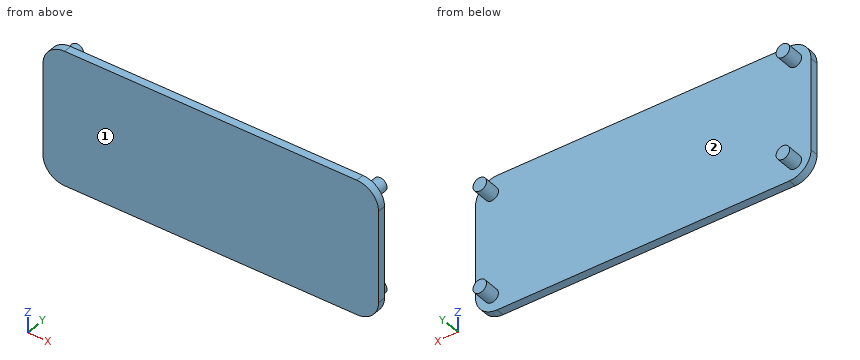
from build123d import *

# Parameters (mm, degrees)
CROQUIS1_W              = 62
CROQUIS1_H              = 25
SALIENTE_EXTRUIR1_DEPTH = 1.5
REDONDEO1_R             = 4
CROQUIS2_R              = 1.25
SALIENTE_EXTRUIR2_DEPTH = 3


with BuildPart() as part:
    # Croquis1 → Saliente-Extruir1 (new body)
    with BuildSketch(Plane(origin=(0, 0, 0), x_dir=(1, 0, 0), z_dir=(0, 1, 0))):
        Rectangle(CROQUIS1_W, CROQUIS1_H)
    extrude(amount=SALIENTE_EXTRUIR1_DEPTH)

    # Redondeo1
    redondeo1_edges = [part.edges().sort_by_distance(p)[0] for p in [
        (31, 0.75, 12.5),
        (-31, 0.75, 12.5),
        (-31, 0.75, -12.5),
        (31, 0.75, -12.5),
    ]]
    fillet(redondeo1_edges, radius=REDONDEO1_R)

    # Croquis2 → Saliente-Extruir2 (add)
    with BuildSketch(Plane(origin=(0, 1.5, 0), x_dir=(1, 0, 0), z_dir=(0, 1, 0))):
        with Locations((-28, 9.47)):
            Circle(CROQUIS2_R)
        with Locations((28, 9.47)):
            Circle(CROQUIS2_R)
        with Locations((28, -9.47)):
            Circle(CROQUIS2_R)
        with Locations((-28, -9.47)):
            Circle(CROQUIS2_R)
    extrude(amount=SALIENTE_EXTRUIR2_DEPTH)


solid = part.part
Model file for the job. Use its own axes, mm. Face numbers are marked on the shaded views. Coordinates: 2 decimals unless noted, no trailing zeros. Order: outer loops, then holes, each group sorted by start corner. A loop starts at its lowest first (then second) coordinate and runs counter-clockwise, first axis right, second up. Notation, with made-up numbers: (57.25, 63.5) -> (75.25, 63.5) arc R29 ccw to (75.25, 83.5) -> close; hole circle Ø8 at (35, -36). An arc over 180 degrees is marked (long way). Return JSON: item names as keys, results as strings. Group by question number.
Item 1: Wall check: line 1 along Y through (x, z) = (27, -4); line 2 along X through (y, z) = (3.8, 9). Give the ranges that are in metal, low to high. Write a range as [from, to].
Item 2: Saw through at A-A on y = 2.5. Write the cut outline in (x, z), then the cut area to 3 significant figures.
Item 3: Flat gauge pins, fed straight in: P1, Ø12.5, axis at x = 12, z = 1, coming from the +Y side; P2, Ø1, axis at y = 4, z = -8, coming from the -X side. Where does each tip first touch, or does it go through?
Item 4: Saw through at C-C on x = 28. Write the cut outline in (y, z), then the cut area to 3 significant figures.
Item 5: Saw through at B-B on z = 9.47. Write the cut outline in (x, y), then the cut area to 3 significant figures.
Item 6: Saw through at D-D on z = -2.75. Write the cut outline in (x, y).
Item 7: Pull direction Y, two halves, no side cores. Call the marked faces 1 and 2: pulls with the +Y half, pulls with the -Y half, needs draft (parallel to the pull), parting line crosses it, or undercut.
Values found:
{
 "1": {"line 1": "y = [0, 1.5]", "line 2": "x = [-29.16, -26.84], [26.84, 29.16]"},
 "2": {"outline": "circle Ø2.5 at (-28, -9.47); circle Ø2.5 at (-28, 9.47); circle Ø2.5 at (28, -9.47); circle Ø2.5 at (28, 9.47)", "area": "19.6 mm2"},
 "3": {"P1": "stops at y = 1.5", "P2": "stops at x = -28.79"},
 "4": {"outline": "(0, -12.37) -> (1.5, -12.37) -> (1.5, -10.72) -> (4.5, -10.72) -> (4.5, -8.22) -> (1.5, -8.22) -> (1.5, 8.22) -> (4.5, 8.22) -> (4.5, 10.72) -> (1.5, 10.72) -> (1.5, 12.37) -> (0, 12.37) -> close", "area": "52.1 mm2"},
 "5": {"outline": "(-30.88, 0) -> (30.88, 0) -> (30.88, 1.5) -> (29.25, 1.5) -> (29.25, 4.5) -> (26.75, 4.5) -> (26.75, 1.5) -> (-26.75, 1.5) -> (-26.75, 4.5) -> (-29.25, 4.5) -> (-29.25, 1.5) -> (-30.88, 1.5) -> close", "area": "108 mm2"},
 "6": {"outline": "(-31, 0) -> (31, 0) -> (31, 1.5) -> (-31, 1.5) -> close"},
 "7": {"face 1": "pulls with the -Y half", "face 2": "pulls with the +Y half"}
}
